For this review, use the dimensioned drawing (mm, ordinates from the lowest corner) and the shaded views. Give positions to 0.01 mm unless a question says otherwise; leave off trailing zeros. Write each loop counter-clockwise with the first axis right and the second up, starting at its lowest first coordinate (ties: lowest second). Pieces come first, ordered by that corner, then holes.
1) We need section B-B on y = 15.75. Give the boundary of the cut face in (x, z).
2) Wall thickness on line 1 along X through (y, z) = (9, 72.5); line 2 along Y through (x, z) = (10, 62.5); line 3 along X through (y, z) = (16.5, 109.5): over which ranges is each line inside the solid? List them lowest first.
3) We need section C-C on z = 22. Give the boundary of the cut face in (x, y).
4) For P1, Ø2, axis at y = 10, z = 30, coming from the -X side; P2, Ø1, axis at x = 2, z = 51.5, coming from the -Y side; P3, Ø5, axis at x = 6, y = 13, coming from the +Z side; P4, Ø6, axis at x = 5.5, z = 74.5, coming from the +Y side, all flat-tipped, find the tip position at first contact; note any pin that passes through.
5) We need section A-A on x = 4. Give the boundary of the cut face in (y, z).
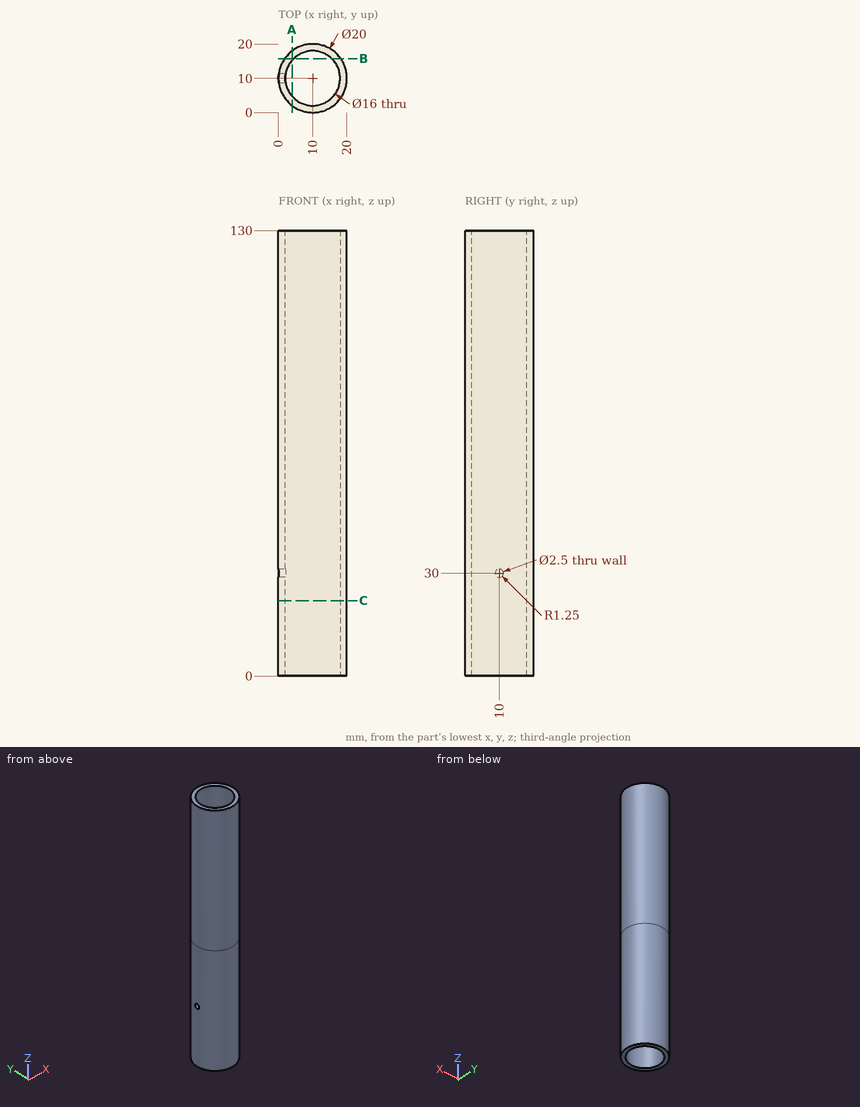
Results list:
1. outline: (1.82, 0) - (4.44, 0) - (4.44, 130) - (1.82, 130) - close; (15.56, 0) - (18.18, 0) - (18.18, 130) - (15.56, 130) - close
2. line 1: x = 0.05 to 2.06, 17.94 to 19.95
2. line 2: y = 0 to 2, 18 to 20
2. line 3: x = 2.4 to 5.34, 14.66 to 17.6
3. outline: circle Ø20 at (10, 10); hole circle Ø16 at (10, 10)
4. P1: stops at x = 17.94
4. P2: stops at y = 3.39
4. P3: passes through
4. P4: stops at y = 19.89
5. outline: (2, 0) - (4.71, 0) - (4.71, 130) - (2, 130) - close; (15.29, 0) - (18, 0) - (18, 130) - (15.29, 130) - close
